CAD build for the part. Positions are in the model's coordinates, mm. A direction names the side the tool comes from. Give positions to 0.01 mm unless a question says otherwise; leave off trailing zeros. Loops run counter-clockwise (first coordinate to the right, second up) from the corner with the lowest first, then second, coordinate; pieces in that order, holes last.
```python
from build123d import *

# Parameters (mm, degrees)
F1_DEPTH = 50.8
F2_W     = 127
F2_H     = 50.8
F3_DEPTH = 76.2
F4_SIZE  = 50.8


with BuildPart() as f1:
    # F0 (on Top) → F1 (new body)
    with BuildSketch(Plane.XY):
        Polygon((-65.568145, 25.4), (-65.568145, -76.2), (61.431855, -76.2), (137.631855, 0), (137.631855, 25.4), align=None)
    extrude(amount=F1_DEPTH)

    # F2 (on face) → F3 (join)
    with BuildSketch(Plane.XY.offset(50.8)):
        with Locations((-2.068145, 0)):
            Rectangle(F2_W, F2_H)
    extrude(amount=F3_DEPTH)

    # F4
    f4_edges = [f1.edges().sort_by_distance(p)[0] for p in [
        (61.431855, 0, 127),
    ]]
    chamfer(f4_edges, length=F4_SIZE)


solid = f1.part
```
1. Saw through at C-C, the plane y = 18. List the corners of the cut face in (x, z).
Responses:
outline: (-65.57, 0) - (137.63, 0) - (137.63, 50.8) - (61.43, 50.8) - (61.43, 76.2) - (10.63, 127) - (-65.57, 127) - close
2. Drop flat-ended pins along their axis: pin 1 (1 mm diameter, centred on x = -44, y = -38.5, fed in from +Z); pin 2 (10 mm diameter, centred on y = 4.5, z = 98, fed in from +X); pin 3 (4 mm diameter, centred on x = 95, y = 10, fed in from -Z); pin 4 (1.5 mm diameter, centred on x = 74.5, z = 24, fed in from -Y). Give the stop position or say it passes through.
Responses:
pin 1: stops at z = 50.8
pin 2: stops at x = 44.63
pin 3: stops at z = 0
pin 4: stops at y = -63.88
3. Saw through at A-A, the plane z = 13.5. List the corners of the cut face in (x, y), and give its area (3 significant figures).
Responses:
outline: (-65.57, -76.2) - (61.43, -76.2) - (137.63, 0) - (137.63, 25.4) - (-65.57, 25.4) - close
area: 17,700 mm2
4. Saw through at B-B, the plane x = 8. List the corners of the cut face in (y, z).
Responses:
outline: (-76.2, 0) - (25.4, 0) - (25.4, 127) - (-25.4, 127) - (-25.4, 50.8) - (-76.2, 50.8) - close
5. Saw through at D-D, the plane y = -11. List the corners of the cut face in (x, z).
Responses:
outline: (-65.57, 0) - (126.63, 0) - (126.63, 50.8) - (61.43, 50.8) - (61.43, 76.2) - (10.63, 127) - (-65.57, 127) - close
6. Tool access for faces 1 (the face through (61.432, 0, 63)), 2 (the face through (-3, -25.4, 88)), 3 (the face through (137.632, 13, 25)): list every direction of +Z, -Z, +X, -X, +Y, -Y with a clear straight run to the whole face (end or side of a thin tool).
Responses:
face 1: +Z, +X, +Y, -Y
face 2: +Z, +X, -X, -Y
face 3: +Z, -Z, +X, +Y, -Y
7. Probe line 1 along Y through (x, z) = (29, 93); line 2 along X through (y, z) = (15, 55.5); line 3 along Z through (x, y) = (26, -64.5). List the from-to ranges inside material, lowest first.
Responses:
line 1: y = -25.4 to 25.4
line 2: x = -65.57 to 61.43
line 3: z = 0 to 50.8
